Here's how the part is built. I have some questions about the finished solid (model axes, mm). A direction names the side the tool comes from. Coordinates: 2 decimals unless noted, no trailing zeros. Write each loop counter-clockwise with the first axis right and the second up, starting at its lowest first coordinate (ties: lowest second). Pieces come first, ordered by that corner, then holes.
Item 1: If we section it at A-A (x = 0): Please give me the cut outline in (y, z).
Item 2: If we section it at C-C (y = -15.75): Please give me the cut outline in (x, z), then the cut area to 3 significant figures.
Item 3: If we section it at B-B (z = 24.5): Please give me the cut outline in (x, y).
Item 4: I'm going to push a flat-ended pin straight in: pin 1 Ø11.5 at (x, z) = (12, 28) entering from -Y. Where does the tip first touch, or does it pass through?
Item 5: We'd pull the mould along X, two halves only. Please class faces 3 (the face through (-7.71, -9.7, 22.47)), 4 (the face through (-7, -10, 44.45)), 5 (the face through (-28.384, -13, 22)): +X half, -X half, draft (parallel to the pull), parting line (faces both ways), or undercut.
Item 6: For faces 1 (the face through (0, 0, 18)), 2 (the face through (-7.104, -18.961, 40.548)), which set-ups out of +Z, -Z, +X, -X, +Y, -Y let a thin tool reach every point of the face, with its end or its side?
Item 7: If I drill on line 1 (Z direction, x = 0, y = -9.25); line 2 (Y direction, x = 14, z = 30); line 3 (Z direction, x = 0, y = -15), over which ranges is the centre line in solid material (lowest first)?
Item 8: If we section it at D-D (z = 41.5): Please give me the cut outline in (x, y).
from build123d import *

# Parameters (mm, degrees)
F0_W     = 57.15
F0_H     = 44.45
F1_DEPTH = 25.4
F2_W     = 38.1
F2_H     = 12.7
F3_DEPTH = 44.45
F5_DEPTH = 12.7
F6_R     = 9.716138
F7_DEPTH = 25.401


with BuildPart() as f1:
    # F0 (on Front) → F1 (new body)
    with BuildSketch(Plane.XZ):
        with Locations((0.191138, 22.225)):
            Rectangle(F0_W, F0_H)
    extrude(amount=F1_DEPTH)

    # F2 (on face) → F3 (cut)
    with BuildSketch(Plane.XY.offset(44.45)):
        with Locations((9.716138, -19.05)):
            Rectangle(F2_W, F2_H)
    extrude(amount=-F3_DEPTH, mode=Mode.SUBTRACT)

    # F4 (on face) → F5 (join)
    with BuildSketch(Plane.XZ.offset(12.7)):
        Polygon((16.066138, 0), (-9.333862, 44.45), (-9.333862, 0), align=None)
    extrude(amount=F5_DEPTH)

    # F6 (on Front) → F7 (cut, through all)
    with BuildSketch(Plane.XZ):
        with Locations((0, 28.383862)):
            Circle(F6_R)
    extrude(amount=F7_DEPTH, mode=Mode.SUBTRACT)


solid = f1.part
Answer list:
1. outline: (-25.4, 0) - (0, 0) - (0, 18.67) - (-25.4, 18.67) - close; (-12.7, 38.1) - (0, 38.1) - (0, 44.45) - (-12.7, 44.45) - close
2. outline: (-28.38, 0) - (16.07, 0) - (4.7, 19.88) arc R9.72 cw to (-4.94, 36.75) - (-9.33, 44.45) - (-28.38, 44.45) - close
2. area: 1,270 mm2
3. outline: (-28.38, -25.4) - (-8.91, -25.4) - (-8.91, 0) - (-28.38, 0) - close; (8.91, -12.7) - (28.77, -12.7) - (28.77, 0) - (8.91, 0) - close
4. pin 1: stops at y = -12.7
5. face 3: undercut
5. face 4: draft
5. face 5: -X half
6. face 1: +Z, -Z, +X, -X, +Y
6. face 2: +Z, +X, -Y
7. line 1: z = 0 to 18.67, 38.1 to 44.45
7. line 2: y = -12.7 to 0
7. line 3: z = 0 to 18.67
8. outline: (-28.38, -25.4) - (-7.65, -25.4) - (-7.65, -12.7) - (28.77, -12.7) - (28.77, 0) - (-28.38, 0) - close
